Read the model definition and answer for the solid it produces. Units are mm, in the model's axes. Face numbers are marked on the shaded views. A direction names the side the tool comes from. Round coordinates to 2 decimals unless told otherwise and drop trailing zeros. Order: outer loops, then holes, each group sorted by start corner. A loop starts at its lowest first (then second) coordinate and runs counter-clockwise, first axis right, second up. Notation, with made-up numbers: (-3, -6) - (11, -6) arc R14 cw to (11, 14) - close; hole circle Ø8 at (-5.5, 40). An arc over 180 degrees is marked (long way). One line per question, with ' | ' between items. Start each with the question number.
1) For the marked faces 5, 6 and 7, determine the directions among +Z, -Z, +X, -X, +Y, -Y from which every point of the face is accessible in a straight line to the end or side of a thin tool.
2) The part is cut by section B-B, the plane y = -15.25. Give the vertices of the cut face in (x, z), plus the area to 3 significant figures.
3) Flat-ended cylindrical pins translate along their axes: pin 1 (10 mm diameter, centred on x = -37, y = -9, fed in from -Z); pin 2 (1 mm diameter, centred on x = -34.5, y = 12.5, fed in from +Z); pin 3 (3.5 mm diameter, centred on x = -52.79, y = 17.36, fed in from -Z); pin 4 (2 mm diameter, centred on x = 7, y = 15.5, fed in from +Z). Find the tip coordinate at first contact, or state that the pin passes through.
4) Straight lines are drawn through the part: line 1 (X direction, y = -10.5, z = 9); line 2 (Z direction, x = -2, y = 17.5); line 3 (Z direction, x = 51, y = -9). For each, find the intervals that lie inside material, in ascending order. Write a range as from..to.
5) The part is cut by section A-A, the plane x = 0. Give the vertices of the cut face in (y, z), plus the area to 3 significant figures.
6) The part is cut by section C-C, the plane z = 41. Give the vertices of the cut face in (x, y), plus the area to 3 significant figures.
7) The mould has two halves that part along X. Classify the marked faces 1, 2, 3 and 4: pulls with the +X half, pulls with the -X half, needs draft (parallel to the pull), parting line crosses it, or undercut.
8) The part is cut by section D-D, the plane y = 10.5. Give the vertices of the cut face in (x, z).
from build123d import *

# Parameters (mm, degrees)
F0_W     = 50
F0_H     = 50
F0_R     = 1.75
F0_R_2   = 12.5
F1_DEPTH = 5
F3_DEPTH = 50
F5_D     = 4.4


with BuildPart() as f1:
    # F0 (on Top) → F1 (new body)
    with BuildSketch(Plane.XY):
        Rectangle(F0_W, F0_H)
        with Locations((-15.25, -15.25)):
            Circle(F0_R, mode=Mode.SUBTRACT)
        with Locations((15.25, -15.25)):
            Circle(F0_R, mode=Mode.SUBTRACT)
        with Locations((-15.25, 15.25)):
            Circle(F0_R, mode=Mode.SUBTRACT)
        Circle(F0_R_2, mode=Mode.SUBTRACT)
        with Locations((15.25, 15.25)):
            Circle(F0_R, mode=Mode.SUBTRACT)
    extrude(amount=F1_DEPTH)

    # F2 (on face) → F3 (join, through all)
    with BuildSketch(Plane.XZ.offset(25)):
        Polygon((-46.7986041229, 39.5), (-25, 0), (-25, 5), (-22.0484650111, 5), (-43.847069134, 44.5), (-61.7379361051, 44.5), (-61.7379361051, 39.5), align=None)
        Polygon((25, 5), (25, 0), (46.7986041229, 39.5), (61.7379361051, 39.5), (61.7379361051, 44.5), (43.847069134, 44.5), (22.0484650111, 5), align=None)
    extrude(amount=-F3_DEPTH)

    # F5 (through all)
    with Locations(Plane.XY.offset(44.5)):
        with Locations((-52.7925026196, 17.3637714833), (-52.7925026196, -18.6362285167), (52.7925026196, -18.6362285167), (52.7925026196, 17.3637714833)):
            Hole(F5_D / 2)


solid = f1.part
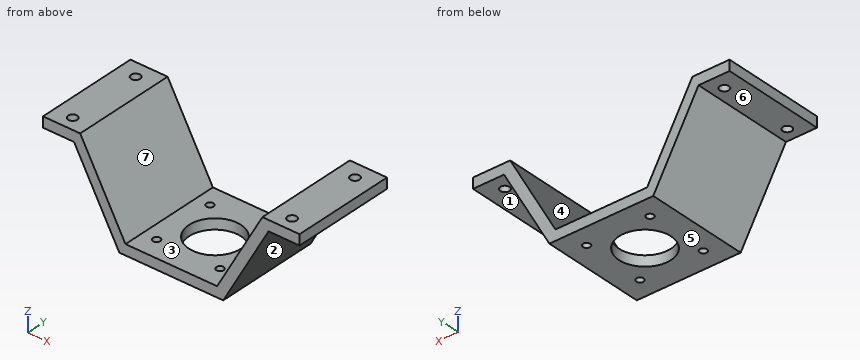
Values:
1) face 5: -Z, +X, -X, +Y, -Y | face 6: -Z, -X, +Y, -Y | face 7: +Z, +Y, -Y
2) outline: (-61.74, 39.5) - (-46.8, 39.5) - (-25, 0) - (-17, 0) - (-17, 5) - (-22.05, 5) - (-43.85, 44.5) - (-61.74, 44.5) - close; (-13.5, 0) - (13.5, 0) - (13.5, 5) - (-13.5, 5) - close; (17, 0) - (25, 0) - (46.8, 39.5) - (61.74, 39.5) - (61.74, 44.5) - (43.85, 44.5) - (22.05, 5) - (17, 5) - close | area: 816 mm^2
3) pin 1: stops at z = 12.68 | pin 2: stops at z = 28.47 | pin 3: passes through | pin 4: stops at z = 5
4) line 1: x = -29.97..-24.26, 24.26..29.97 | line 2: z = 0..5 | line 3: z = 39.5..44.5
5) outline: (-25, 0) - (-12.5, 0) - (-12.5, 5) - (-25, 5) - close; (12.5, 0) - (25, 0) - (25, 5) - (12.5, 5) - close | area: 125 mm^2
6) outline: (-61.74, -25) - (-41.92, -25) - (-41.92, 25) - (-61.74, 25) - close; (41.92, -25) - (61.74, -25) - (61.74, 25) - (41.92, 25) - close; hole circle Ø4.4 at (-52.79, -18.64); hole circle Ø4.4 at (-52.79, 17.36); hole circle Ø4.4 at (52.79, -18.64); hole circle Ø4.4 at (52.79, 17.36) | area: 1,920 mm^2
7) face 1: needs draft | face 2: pulls with the +X half | face 3: undercut | face 4: undercut
8) outline: (-61.74, 39.5) - (-46.8, 39.5) - (-25, 0) - (-6.78, 0) - (-6.78, 5) - (-22.05, 5) - (-43.85, 44.5) - (-61.74, 44.5) - close; (6.78, 0) - (25, 0) - (46.8, 39.5) - (61.74, 39.5) - (61.74, 44.5) - (43.85, 44.5) - (22.05, 5) - (6.78, 5) - close
